```python
from build123d import *

# Parameters (mm, degrees)
SKETCH2_W                = 10
SKETCH2_H                = 80
BOSS_EXTRUDE1_DEPTH      = 10
FILLET1_R                = 5
CUT_EXTRUDE1_DEPTH       = 3
CUT_EXTRUDE2_START       = 7
SKETCH3_2_W              = 10
SKETCH3_2_H              = 9
CUT_EXTRUDE2_DEPTH       = 3
CUT_EXTRUDE4_START       = -4
CUT_EXTRUDE4_DEPTH       = 46.533119315
SKETCH7_R                = 1.5
CUT_EXTRUDE5_DEPTH       = 41.914545091
BOSS_EXTRUDE2_DEPTH      = 7
BOSS_EXTRUDE2_DEPTH_BACK = 7
SKETCH9_W                = 15
SKETCH9_H                = 50
FILLET3_R                = 7


with BuildPart() as part:
    # Sketch2 → Boss-Extrude1 (new body)
    with BuildSketch(Plane.XY):
        Rectangle(SKETCH2_W, SKETCH2_H)
    extrude(amount=BOSS_EXTRUDE1_DEPTH)

    # Fillet1
    fillet1_edges = [part.edges().sort_by_distance(p)[0] for p in [
        (-5, 0, 0),
        (5, 0, 0),
        (5, 0, 10),
        (-5, 0, 10),
    ]]
    fillet(fillet1_edges, radius=FILLET1_R - 0.0001)  # a hair under: the kernel refuses the full size

    # Sketch3 → Cut-Extrude1 (cut)
    with BuildSketch(Plane.XY):
        with BuildLine():
            Line((-5, -31), (-4.5, -35.5))
            ThreePointArc((-4.5, -35.5), (0, -40), (4.5, -35.5))
            Line((4.5, -35.5), (5, -31))
            Line((5, -31), (-5, -31))
        make_face()
        with BuildLine():
            Line((0, -40), (5, -40))
            Line((5, -40), (5, -31))
            Line((5, -31), (4.5, -35.5))
            ThreePointArc((4.5, -35.5), (3.181980515, -38.681980515), (0, -40))
        make_face()
        with BuildLine():
            Line((-5, -40), (0, -40))
            ThreePointArc((0, -40), (-3.181980515, -38.681980515), (-4.5, -35.5))
            Line((-4.5, -35.5), (-5, -31))
            Line((-5, -31), (-5, -40))
        make_face()
    cut_extrude1 = extrude(amount=CUT_EXTRUDE1_DEPTH, mode=Mode.SUBTRACT)

    # Sketch3<2> → Cut-Extrude2 (cut)
    with BuildSketch(Plane.XY.offset(CUT_EXTRUDE2_START)):
        with Locations((0, -35.5)):
            Rectangle(SKETCH3_2_W, SKETCH3_2_H)
    cut_extrude2 = extrude(amount=CUT_EXTRUDE2_DEPTH, mode=Mode.SUBTRACT)

    # Mirror1: Cut-Extrude1, Cut-Extrude2 across plane
    add(cut_extrude1.mirror(Plane.ZX), mode=Mode.SUBTRACT)
    add(cut_extrude2.mirror(Plane.ZX), mode=Mode.SUBTRACT)

    # Sketch3<4> → Cut-Extrude4 (cut)
    with BuildSketch(Plane.XY.offset(CUT_EXTRUDE4_START)):
        with BuildLine():
            Line((0, -40), (5, -40))
            Line((5, -40), (5, -31))
            Line((5, -31), (4.5, -35.5))
            ThreePointArc((4.5, -35.5), (3.181980515, -38.681980515), (0, -40))
        make_face()
        with BuildLine():
            Line((-5, -40), (0, -40))
            ThreePointArc((0, -40), (-3.181980515, -38.681980515), (-4.5, -35.5))
            Line((-4.5, -35.5), (-5, -31))
            Line((-5, -31), (-5, -40))
        make_face()
    cut_extrude4 = extrude(amount=CUT_EXTRUDE4_DEPTH, mode=Mode.SUBTRACT)

    # Sketch7 → Cut-Extrude5 (cut, through all)
    with BuildSketch(Plane(origin=(0, 0, 3), x_dir=(-1, 0, 0), z_dir=(0, 0, -1))):
        with Locations((0, -35.5)):
            Circle(SKETCH7_R)
    cut_extrude5 = extrude(amount=-CUT_EXTRUDE5_DEPTH, mode=Mode.SUBTRACT)

    # Mirror3: Cut-Extrude5 across plane
    add(cut_extrude5.mirror(Plane.ZX), mode=Mode.SUBTRACT)

    # Mirror4: Cut-Extrude4 across plane
    add(cut_extrude4.mirror(Plane.ZX), mode=Mode.SUBTRACT)

    # Sketch9 → Boss-Extrude2 (add, two sides: drawn at the far end of the back side and taken through both)
    with BuildSketch(Plane.XY.offset(5).offset(-BOSS_EXTRUDE2_DEPTH_BACK)):
        Rectangle(SKETCH9_W, SKETCH9_H)
    extrude(amount=BOSS_EXTRUDE2_DEPTH + BOSS_EXTRUDE2_DEPTH_BACK)

    # Fillet3
    fillet3_edges = [part.edges().sort_by_distance(p)[0] for p in [
        (-7.5, 0, 12),
        (7.5, 0, 12),
        (7.5, 0, -2),
        (-7.5, 0, -2),
    ]]
    fillet(fillet3_edges, radius=FILLET3_R - 0.0001)  # a hair under: the kernel refuses the full size


solid = part.part
```
Model file for the job. Use its own axes, mm. A direction names the side the tool comes from. Coordinates: 2 decimals unless noted, no trailing zeros. Loops run counter-clockwise (first coordinate to the right, second up) from the corner with the lowest first, then second, coordinate; pieces in that order, holes last. Notation, with made-up numbers: (-29, -23.5) -> (-7, -23.5) arc R25 ccw to (-7, -6.5) -> close; hole circle Ø3 at (-26.5, 55.5). An arc over 180 degrees is marked (long way). Answer as a JSON object with one key per item and string values.
Q1. Flat gauge pins, fed straight in: P1, Ø1.5, axis at x = -5, y = 30, coming from the -Z side; P2, Ø4, axis at x = 0, y = -35.5, coming from the +Z side; P3, Ø4.5, axis at x = -2, y = -33.5, coming from the -Z side. Where does each tip first touch, or does it go through?
Report:
{"P1": "stops at z = 2.37", "P2": "stops at z = 7", "P3": "stops at z = 3"}
Q2. Cut at B-B (z = 6). List the corners of the cut face in (x, y), and give its area (3 significant figures).
Report:
{"outline": "(-7.43, -25) -> (-4.9, -25) -> (-4.9, -31.91) -> (-4.5, -35.5) arc R4.5 ccw to (4.5, -35.5) -> (4.9, -31.91) -> (4.9, -25) -> (7.43, -25) -> (7.43, 25) -> (4.9, 25) -> (4.9, 31.91) -> (4.5, 35.5) arc R4.5 ccw to (-4.5, 35.5) -> (-4.9, 31.91) -> (-4.9, 25) -> (-7.43, 25) -> close; hole circle Ø3 at (0, -35.5); hole circle Ø3 at (0, 35.5)", "area": "995 mm2"}
Q3. 3-axis set-ups, long thin cutter, end or side, ignore diameter. For faces 4 (the flat face through (0, 31, 8)), 5 (the flat face through (-1, -34, 7)), 6 (the flat face through (0, 31, 2)), 7 (the flat face through (2, -25, 0)), 8 (the flat face through (2, 25, 0)): which of +Z, -Z, +X, -X, +Y, -Y reach the whole face in a straight line?
Report:
{"face 4": "+Z, +X, -X, +Y", "face 5": "+Z, +X, -X, -Y", "face 6": "-Z, +X, -X, +Y", "face 7": "-Y", "face 8": "+Y"}
Q4. Pull direction Y, two halves, no side cores. Call faces 1 (the cylindrical face through (0, 37, 5)), 2 (the cylindrical face through (-4, -29, 8)), 3 (the flat face through (0, -31, 8)): released by +Y, released by -Y, zero draft, split by the parting line, or undercut.
Report:
{"face 1": "undercut", "face 2": "zero draft", "face 3": "released by -Y"}
Q5. Probe probe 1 along Y at (x, z) = (0, 4.2); probe 2 along X at (y, z) = (35.5, 5.5); probe 3 along Y at (x, z) = (5.5, 9.5). List the from-to ranges inside material, lowest first.
Report:
{"probe 1": "y = -40 to -37, -34 to 34, 37 to 40", "probe 2": "x = -4.5 to -1.5, 1.5 to 4.5", "probe 3": "y = -25 to 25"}
Q6. Cut at C-C (z = 1.25). List the corners of the cut face in (x, y), and give its area (3 significant figures).
Report:
{"outline": "(-6.41, -25) -> (-3.31, -25) -> (-3.31, -31) -> (3.31, -31) -> (3.31, -25) -> (6.41, -25) -> (6.41, 25) -> (3.31, 25) -> (3.31, 31) -> (-3.31, 31) -> (-3.31, 25) -> (-6.41, 25) -> close", "area": "720 mm2"}
